Design review of the part built by this model. Coordinates are the model's own, in mm. Face numbers are marked on the shaded views. A direction names the side the tool comes from. Give positions to 0.01 mm unless a question says otherwise; leave off trailing zeros. Order: outer loops, then holes, each group sorted by start corner. A loop starts at its lowest first (then second) coordinate and runs counter-clockwise, first axis right, second up.
```python
from build123d import *

# Parameters (mm, degrees)
CROQUIS1_R              = 10
SALIENTE_EXTRUIR1_DEPTH = 22.5
CROQUIS3_R              = 2.65
SALIENTE_EXTRUIR2_DEPTH = 6
CROQUIS5_R              = 5
CORTAR_EXTRUIR1_DEPTH   = 1
SALIENTE_EXTRUIR3_DEPTH = 20
CROQUIS8_R              = 10
CORTAR_EXTRUIR2_DEPTH   = 45
SALIENTE_EXTRUIR4_DEPTH = 2.5
CROQUIS15_W             = 31.132875884
CROQUIS15_H             = 39.860662673
CORTAR_EXTRUIR3_DEPTH   = 6


with BuildPart() as part:
    # Croquis1 → Saliente-Extruir1 (new body, symmetric)
    with BuildSketch(Plane(origin=(0, 0, 0), x_dir=(0, 0, -1), z_dir=(1, 0, 0))):
        with BuildLine():
            Line((-20, -24), (20, -24))
            Line((20, -24), (20, 0))
            ThreePointArc((20, 0), (0, 20), (-20, 0))
            Line((-20, 0), (-20, -24))
        make_face()
        Circle(CROQUIS1_R, mode=Mode.SUBTRACT)
    extrude(amount=SALIENTE_EXTRUIR1_DEPTH, both=True)

    # Croquis3 → Saliente-Extruir2 (add)
    with BuildSketch(Plane(origin=(0, -24, 0), x_dir=(-1, 0, 0), z_dir=(0, -1, 0))):
        with BuildLine():
            Line((22.5, 30), (22.5, 18.749800444))
            Line((22.5, 18.749800444), (22.5, -30))
            ThreePointArc((22.5, -30), (20.303300859, -35.303300859), (15, -37.5))
            Line((15, -37.5), (-15, -37.5))
            ThreePointArc((-15, -37.5), (-20.303300859, -35.303300859), (-22.5, -30))
            Line((-22.5, -30), (-22.5, 30))
            ThreePointArc((-22.5, 30), (-20.303300859, 35.303300859), (-15, 37.5))
            Line((-15, 37.5), (15, 37.5))
            ThreePointArc((15, 37.5), (20.303300859, 35.303300859), (22.5, 30))
        make_face()
        with Locations((15, 30)):
            Circle(CROQUIS3_R, mode=Mode.SUBTRACT)
        with Locations((-15, 30)):
            Circle(CROQUIS3_R, mode=Mode.SUBTRACT)
        with Locations((15, -30)):
            Circle(CROQUIS3_R, mode=Mode.SUBTRACT)
        with Locations((-15, -30)):
            Circle(CROQUIS3_R, mode=Mode.SUBTRACT)
    extrude(amount=SALIENTE_EXTRUIR2_DEPTH)

    # Croquis5 → Cortar-Extruir1 (cut)
    with BuildSketch(Plane(origin=(0, -24, 0), x_dir=(-1, 0, 0), z_dir=(0, -1, 0))):
        with Locations((15, 30)):
            Circle(CROQUIS5_R)
        with Locations((-15, 30)):
            Circle(CROQUIS5_R)
        with Locations((15, -30)):
            Circle(CROQUIS5_R)
        with Locations((-15, -30)):
            Circle(CROQUIS5_R)
    extrude(amount=CORTAR_EXTRUIR1_DEPTH, mode=Mode.SUBTRACT)

    # Croquis6 → Saliente-Extruir3 (add, symmetric)
    with BuildSketch(Plane.XY):
        Polygon((-15, 20.067860351), (-15, 32), (-32.5, 32), (-32.5, 26), (-26.787274513, 26), (-26.787274513, 20), (-32.5, 20), (-32.5, 14), (-22.5, 14), (-22.5, 0), (-15, 0), align=None)
    extrude(amount=SALIENTE_EXTRUIR3_DEPTH, both=True)

    # Croquis8 → Cortar-Extruir2 (cut)
    with BuildSketch(Plane.ZY.offset(22.5)):
        Circle(CROQUIS8_R)
    extrude(amount=-CORTAR_EXTRUIR2_DEPTH, mode=Mode.SUBTRACT)

    # Croquis10 → Saliente-Extruir4 (add, symmetric)
    with BuildSketch(Plane(origin=(0, 0, 0), x_dir=(0, 0, -1), z_dir=(1, 0, 0))):
        Polygon((-18.138791867, 5.125023494), (-37.598536218, -24.265305437), (-18.138791867, -24.265305437), align=None)
        Polygon((37.025889105, -24.265305437), (19.948399075, -24.265305437), (19.948399075, 5.125023494), align=None)
    extrude(amount=SALIENTE_EXTRUIR4_DEPTH, both=True)

    # Croquis15 → Cortar-Extruir3 (cut)
    with BuildSketch(Plane.XZ.offset(30)):
        with Locations((1.933562058, 0.121457578)):
            Rectangle(CROQUIS15_W, CROQUIS15_H)
    extrude(amount=-CORTAR_EXTRUIR3_DEPTH, mode=Mode.SUBTRACT)


solid = part.part
```
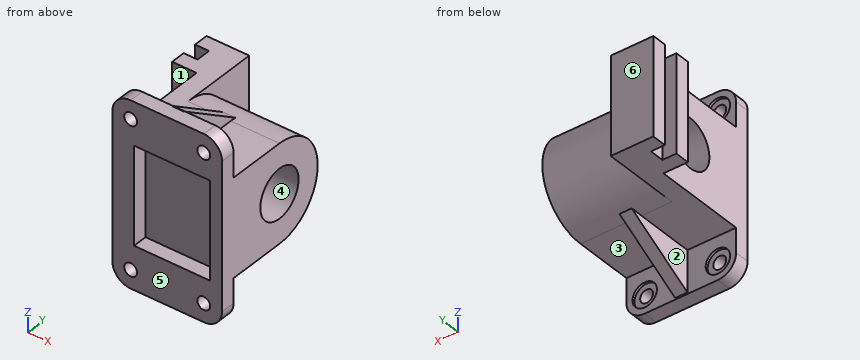
1. For line 1 along Z through (x, y) = (15, -24.3); line 2 along X through (y, z) = (-24.7, 30); line 3 along Z through (x, y) = (-15, -26), list the stretches that pass through material, from the lowest coordinate up.
Recorded:
line 1: z = -37.5 to -35, -25 to -19.81, 20.05 to 25, 35 to 37.5
line 2: x = -22.5 to -20, -10 to 10, 20 to 22.5
line 3: z = -37.5 to -32.65, -27.35 to 27.35, 32.65 to 37.5
2. Take a section at B-B (y = -1). State the section outline as (x, z) points, then the cut area to 3 significant figures.
Recorded:
outline: (-22.5, -20) - (-2.5, -20) - (-2.5, -23.51) - (2.5, -23.51) - (2.5, -20) - (22.5, -20) - (22.5, -9.95) - (-22.5, -9.95) - close; (-22.5, 9.95) - (22.5, 9.95) - (22.5, 20) - (2.5, 20) - (2.5, 22.19) - (-2.5, 22.19) - (-2.5, 20) - (-22.5, 20) - close
area: 933 mm2
3. Take a section at C-C (z = -16). State the section outline as (x, y) points.
Recorded:
outline: (-32.5, 14) - (-22.5, 14) - (-22.5, -30) - (-13.63, -30) - (-13.63, -24) - (17.5, -24) - (17.5, -30) - (22.5, -30) - (22.5, 12) - (-15, 12) - (-15, 32) - (-32.5, 32) - (-32.5, 26) - (-26.79, 26) - (-26.79, 20) - (-32.5, 20) - close
4. Take a section at D-D (y = -11). State the section outline as (x, z) points.
Recorded:
outline: (-22.5, -20) - (-2.5, -20) - (-2.5, -29.32) - (2.5, -29.32) - (2.5, -20) - (22.5, -20) - (22.5, 20) - (2.5, 20) - (2.5, 28.82) - (-2.5, 28.82) - (-2.5, 20) - (-22.5, 20) - close
5. Machinability: for the marked faces 1, 2 and 3, which of the approach directions +Z, -Z, +X, -X, +Y, -Y give a long, thin tool a straight path to every point of the face, cutting with its end or side? Answer none if there is none.
Recorded:
face 1: +Z, -Z, -X, -Y
face 2: -Z, -X, +Y
face 3: -Z, +X, +Y
6. Draft analysis for pull direction Y (two halves, no side actions). For the marked faces 4, 5 and 6, state which applies: pulls with the +Y half, pulls with the -Y half, needs draft (parallel to the pull), parting line crosses it, or undercut.
Recorded:
face 4: undercut
face 5: pulls with the -Y half
face 6: pulls with the +Y half
7. Take a section at A-A (z = 0). State the section outline as (x, y) points.
Recorded:
outline: (-32.5, 14) - (-22.5, 14) - (-22.5, 10) - (22.5, 10) - (22.5, 20) - (-15, 20) - (-15, 32) - (-32.5, 32) - (-32.5, 26) - (-26.79, 26) - (-26.79, 20) - (-32.5, 20) - close; (-22.5, -30) - (-13.63, -30) - (-13.63, -24) - (17.5, -24) - (17.5, -30) - (22.5, -30) - (22.5, -10) - (-22.5, -10) - close
8. For pin 1 (1.5 mm diameter, centred on x = -14.5, y = -24, fed in from +Z); pin 2 (6 mm diameter, centred on x = -15, z = -30, fed in from +Y); pin 3 (1 mm diameter, centred on x = 8, y = 18.5, fed in from -Z), all flat-tipped, find the tip position at first contact; note any pin that passes through.
Recorded:
pin 1: stops at z = 37.5
pin 2: stops at y = -25
pin 3: stops at z = -8.72
